from build123d import *

# Parameters (mm, degrees)
BOSS_EXTRUDE1_DEPTH = 2
SKETCH2_R           = 1
CUT_EXTRUDE1_DEPTH  = 133.597605559
CHAMFER1_SIZE       = 1.5
SKETCH3_W           = 15.5
SKETCH3_H           = 4.5
CUT_EXTRUDE2_DEPTH  = 133.597605559
SKETCH4_W           = 8
SKETCH4_H           = 40
CUT_EXTRUDE3_DEPTH  = 1.3


with BuildPart() as part:
    # Sketch1 → Boss-Extrude1 (new body)
    with BuildSketch(Plane(origin=(0, 0, 0), x_dir=(1, 0, 0), z_dir=(0, 1, 0))):
        Polygon((-74.75, -93.75), (-70.25, -93.75), (-70.25, -91.75), (-14.75, -91.75), (-14.75, -93.75), (4.75, -93.75), (4.75, -91.75), (60.25, -91.75), (60.25, -93.75), (64.75, -93.75), (64.75, -91.75), (91.75, -91.75), (91.75, -87.65), (86.75, -87.65), (86.75, -77.15), (91.75, -77.15), (91.75, 91.75), (18.65, 91.75), (18.65, 83.15), (-28.65, 83.15), (-28.65, 91.75), (-91.75, 91.75), (-91.75, -80.05), (-93.75, -80.05), (-93.75, -84.75), (-91.75, -84.75), (-91.75, -91.75), (-74.75, -91.75), align=None)
    extrude(amount=BOSS_EXTRUDE1_DEPTH)

    # Sketch2 → Cut-Extrude1 (cut, through all)
    with BuildSketch(Plane.XZ):
        with Locations(Location((75, -75, 0), (0, 0, 270))):
            Circle(SKETCH2_R)
        with Locations(Location((-75, -75, 0), (0, 0, 270))):
            Circle(SKETCH2_R)
        with Locations(Location((-75, 75, 0), (0, 0, 270))):
            Circle(SKETCH2_R)
        with Locations(Location((75, 75, 0), (0, 0, 270))):
            Circle(SKETCH2_R)
        with Locations(Location((33.5, 38.5, 0), (0, 0, 270))):
            Circle(SKETCH2_R)
        with Locations(Location((-43.5, 38.5, 0), (0, 0, 270))):
            Circle(SKETCH2_R)
        with Locations(Location((-43.5, -38.5, 0), (0, 0, 270))):
            Circle(SKETCH2_R)
        with Locations(Location((33.5, -38.5, 0), (0, 0, 270))):
            Circle(SKETCH2_R)
    extrude(amount=-CUT_EXTRUDE1_DEPTH, mode=Mode.SUBTRACT)

    # Chamfer1
    chamfer1_edges = [part.edges().sort_by_distance(p)[0] for p in [
        (-75, 2, -74),
        (-75, 2, 76),
        (75, 2, 76),
        (33.5, 2, 39.5),
        (-43.5, 2, 39.5),
        (-43.5, 2, -37.5),
        (33.5, 2, -37.5),
        (75, 2, -74),
    ]]
    chamfer(chamfer1_edges, length=CHAMFER1_SIZE)

    # Sketch3 → Cut-Extrude2 (cut, through all)
    with BuildSketch(Plane.XZ):
        with Locations((-58.5, -87.5)):
            Rectangle(SKETCH3_W, SKETCH3_H)
    extrude(amount=-CUT_EXTRUDE2_DEPTH, mode=Mode.SUBTRACT)

    # Sketch4 → Cut-Extrude3 (cut)
    with BuildSketch(Plane.XZ):
        with Locations((-43.75, -0.25)):
            Rectangle(SKETCH4_W, SKETCH4_H)
    extrude(amount=-CUT_EXTRUDE3_DEPTH, mode=Mode.SUBTRACT)


solid = part.part
Input: part model. Units: mm. Frame: model coordinates. Round coordinates to 2 decimals unless told otherwise and drop trailing zeros. Write each loop counter-clockwise with the first axis right and the second up, starting at its lowest first coordinate (ties: lowest second). Pieces come first, ordered by that corner, then holes.
1) Contact query for flat-ended pins moving along their axis: P1, Ø0.6, axis at y = 1, z = 92.5, coming from the -X side; P2, Ø1.2, axis at x = -75, z = -75, coming from the -Y side; P3, Ø0.6, axis at x = -93, y = 0.5, coming from the -Z side; P4, Ø1, axis at x = 57.5, y = 1, coming from the +Z side. Output: stop coordinate, or through.
2) Draft query along Z for faces 1 (the flat face through (-2, 0, 0)), 2 (the flat face through (-44, 1.3, 0)). Return one class per face: pulls with the +Z half, pulls with the -Z half, needs draft (parallel to the pull), parting line crosses it, or undercut.
3) Cut plane A-A (z = 7.5). Return the cut outline in (x, y).
4) Ray query, L1, parallel to X at y = 0.35, z = -38.5; L2, parallel to X at y = 0.9, z = -6.5; L3, parallel to Z at x = -75, y = 0.3. Return the intervals inside material, ascending.
Geometry says:
1. P1: stops at x = -74.75
1. P2: passes through
1. P3: stops at z = 80.05
1. P4: stops at z = 91.75
2. face 1: needs draft
2. face 2: undercut
3. outline: (-91.75, 0) - (-47.75, 0) - (-47.75, 1.3) - (-39.75, 1.3) - (-39.75, 0) - (91.75, 0) - (91.75, 2) - (-91.75, 2) - close
4. L1: x = -91.75 to -44.5, -42.5 to 32.5, 34.5 to 91.75
4. L2: x = -91.75 to -47.75, -39.75 to 91.75
4. L3: z = -91.75 to -76, -74 to 74, 76 to 91.75
